from build123d import *

# Parameters (mm, degrees)
LINEAR_AUSTRAGEN1_DEPTH              = 473.5
M8_GEWINDEBOHRUNG1_D                 = 6.8
M8_GEWINDEBOHRUNG1_CSINK_D           = 8.05
M8_GEWINDEBOHRUNG1_CSINK_ANGLE       = 90
SCHNITT_LINEAR_AUSTRAGEN2_DEPTH      = 20
FASE1_SIZE                           = 20
F_14_0_14_DURCHMESSER_BOHRUNG1_D     = 14
F_14_0_14_DURCHMESSER_BOHRUNG1_DEPTH = 20
F_14_0_14_DURCHMESSER_BOHRUNG1_TIP   = 4.206024333
F_14_0_14_DURCHMESSER_BOHRUNG2_D     = 14
F_14_0_14_DURCHMESSER_BOHRUNG2_DEPTH = 20
F_14_0_14_DURCHMESSER_BOHRUNG2_TIP   = 4.206024333


with BuildPart() as part:
    # Skizze1 → Linear austragen1 (new, symmetric)
    with BuildSketch(Plane.XY):
        Polygon((8, 28), (8, 23), (55, 23), (55, -12), (-15, -12), (-15, 28), align=None)
    extrude(amount=LINEAR_AUSTRAGEN1_DEPTH, both=True)

    # M8 Gewindebohrung1 (through all)
    with Locations(Plane(origin=(0, 23, 0), x_dir=(-1, 0, 0), z_dir=(0, 1, 0))):
        with Locations((-33, 452.5), (-33, -52.5), (-33, 252.5), (-33, -252.5), (-33, 52.5), (-33, -452.5)):
            CounterSinkHole(M8_GEWINDEBOHRUNG1_D / 2, M8_GEWINDEBOHRUNG1_CSINK_D / 2, counter_sink_angle=M8_GEWINDEBOHRUNG1_CSINK_ANGLE)

    # Skizze20 → Schnitt-Linear austragen2 (cut)
    with BuildSketch(Plane.XZ.offset(12)):
        with BuildLine():
            Line((55, 473.5), (15, 473.5))
            Line((15, 473.5), (15, 373.5))
            Line((15, 373.5), (11, 373.5))
            ThreePointArc((11, 373.5), (-3.849242405, 367.349242405), (-10, 352.5))
            Line((-10, 352.5), (-10, -352.5))
            ThreePointArc((-10, -352.5), (-3.849242405, -367.349242405), (11, -373.5))
            Line((11, -373.5), (15, -373.5))
            Line((15, -373.5), (15, -473.5))
            Line((15, -473.5), (55, -473.5))
            Line((55, -473.5), (55, 473.5))
        make_face()
    extrude(amount=-SCHNITT_LINEAR_AUSTRAGEN2_DEPTH, mode=Mode.SUBTRACT)

    # Fase1
    fase1_edges = [part.edges().sort_by_distance(p)[0] for p in [
        (-15, 28, 0),
    ]]
    chamfer(fase1_edges, length=FASE1_SIZE)

    # Ø14.0 (14) Durchmesser Bohrung1
    with Locations(Plane.XY.offset(473.5)):
        with Locations((0, 0)):
            Hole(F_14_0_14_DURCHMESSER_BOHRUNG1_D / 2, depth=F_14_0_14_DURCHMESSER_BOHRUNG1_DEPTH)
            with Locations((0, 0, -(F_14_0_14_DURCHMESSER_BOHRUNG1_DEPTH + F_14_0_14_DURCHMESSER_BOHRUNG1_TIP / 2))):  # 118° drill point
                Cone(0, F_14_0_14_DURCHMESSER_BOHRUNG1_D / 2, F_14_0_14_DURCHMESSER_BOHRUNG1_TIP, mode=Mode.SUBTRACT)

    # Ø14.0 (14) Durchmesser Bohrung2
    with Locations(Plane(origin=(0, 0, -473.5), x_dir=(-1, 0, 0), z_dir=(0, 0, -1))):
        with Locations((0, 0)):
            Hole(F_14_0_14_DURCHMESSER_BOHRUNG2_D / 2, depth=F_14_0_14_DURCHMESSER_BOHRUNG2_DEPTH)
            with Locations((0, 0, -(F_14_0_14_DURCHMESSER_BOHRUNG2_DEPTH + F_14_0_14_DURCHMESSER_BOHRUNG2_TIP / 2))):  # 118° drill point
                Cone(0, F_14_0_14_DURCHMESSER_BOHRUNG2_D / 2, F_14_0_14_DURCHMESSER_BOHRUNG2_TIP, mode=Mode.SUBTRACT)


solid = part.part
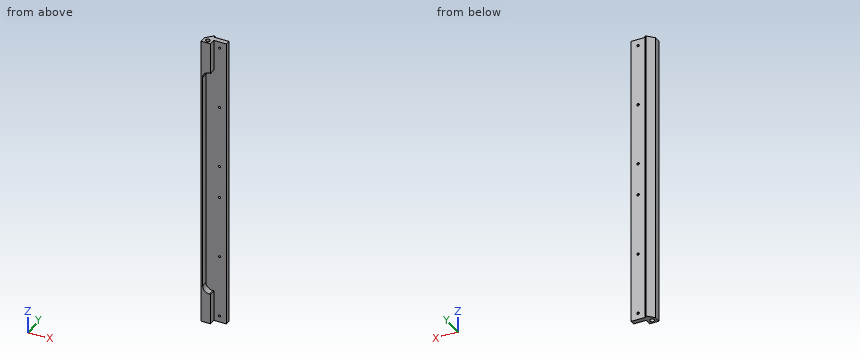
Here's how the part is built. I have some questions about the finished solid (model axes, mm). Coordinates: 2 decimals unless noted, no trailing zeros. Loops run counter-clockwise (first coordinate to the right, second up) from the corner with the lowest first, then second, coordinate; pieces in that order, holes last. Notation, with made-up numbers: (21, 47) -> (59, 47) arc R29 cw to (59, 67) -> close; hole circle Ø7 at (81, 71.5). An arc over 180 degrees is marked (long way). Use one line per item in the form item = value. Start each with the question number.
(1) Please list where these lines run through material, in increasing order: line 1 along X through (y, z) = (0, 464); line 2 along Y through (x, z) = (0, 462.75); line 3 along X through (y, z) = (-9.5, -338).
(2) If we section it at A-A (z = 18.5): Please give me the cut outline in (x, y).
(3) Will these pins go through, and if not, where does the flat tip stop? pin 1 (11 mm diameter, centred on x = 33, z = 52.5, fed in from +Y); pin 2 (1.5 mm diameter, centred on y = 24.5, z = 171.5, fed in from +X); pin 3 (11 mm diameter, centred on x = 33, z = -52.5, fed in from -Y).
(4) If we section it at B-B (z = -401.5): Please give me the cut outline in (x, y), then the cut area to 4 significant figures.
Verdict:
q1.line_1 = -15 to -7, 7 to 15
q1.line_2 = -12 to -7, 7 to 23
q1.line_3 = -15 to -10
q2.outline = (-15, -12) -> (-10, -12) -> (-10, 8) -> (55, 8) -> (55, 23) -> (8, 23) -> (8, 28) -> (5, 28) -> (-15, 8) -> close
q3.pin_1 = 23
q3.pin_2 = 8
q3.pin_3 = 8
q4.outline = (-15, -12) -> (15, -12) -> (15, 8) -> (55, 8) -> (55, 23) -> (8, 23) -> (8, 28) -> (5, 28) -> (-15, 8) -> close
q4.area = 1,565 mm²
